For this review, take the finished solid that the model builds, in its own axes (mm). A direction names the side the tool comes from. Give positions to 0.01 mm unless a question says otherwise; leave off trailing zeros. Loops run counter-clockwise (first coordinate to the right, second up) from the corner with the lowest first, then second, coordinate; pieces in that order, holes last.
```python
from build123d import *

# Parameters (mm, degrees)
F0_W     = 12.7
F0_H     = 12.7
F1_DEPTH = 12.7
F2_DEPTH = 25.4
F3_W     = 12.9194361269
F3_H     = 12.7
F4_DEPTH = 12.7
F5_W     = 12.7
F5_H     = 12.7
F6_DEPTH = 12.7
F7_W     = 12.7
F7_H     = 12.7
F8_DEPTH = 12.7
F9_T     = -2.54


with BuildPart() as f1:
    # F0 (on Front) → F1 (new body)
    with BuildSketch(Plane.XZ):
        with Locations((0.4788246006, 3.6696097578)):
            Rectangle(F0_W, F0_H)
    extrude(amount=F1_DEPTH)

    # F2 (add): a face of the model
    f2_faces = [f1.faces().sort_by_distance(p)[0] for p in [
        (6.8288246006, -6.35, 3.6696097578),
    ]]
    extrude(f2_faces, amount=F2_DEPTH)

    # F3 (on face) → F4 (join)
    with BuildSketch(Plane(origin=(0, 0, 0), x_dir=(-1, 0, 0), z_dir=(0, 1, 0))):
        with Locations((-25.7691065371, 3.6696097578)):
            Rectangle(F3_W, F3_H)
    extrude(amount=F4_DEPTH)

    # F5 (on face) → F6 (join)
    with BuildSketch(Plane(origin=(0, 0, 0), x_dir=(-1, 0, 0), z_dir=(0, 1, 0))):
        with Locations((-0.4788246006, 3.6696097578)):
            Rectangle(F5_W, F5_H)
    extrude(amount=F6_DEPTH)

    # F7 (on face) → F8 (join)
    with BuildSketch(Plane.XY.offset(10.0196097578)):
        with Locations((0.4788246006, -6.35)):
            Rectangle(F7_W, F7_H)
    extrude(amount=F8_DEPTH)

    # F9 (hollow: no face is removed)
    offset(amount=F9_T, kind=Kind.INTERSECTION, mode=Mode.SUBTRACT)


solid = f1.part
```
Item 1: Take a section at B-B on z = 17.5. Give the boundary of the cut face in (x, y), and give its area (3 significant figures).
Answer:
outline: (-5.87, -12.7) - (6.83, -12.7) - (6.83, 0) - (-5.87, 0) - close; hole (-3.33, -10.16) - (4.29, -10.16) - (4.29, -2.54) - (-3.33, -2.54) - close
area: 103 mm2
Item 2: Clearance check with flat-ended pins moving along their axes: pin 1 Ø3.5 at (x, z) = (15, 1) entering from +Y; pin 2 Ø4 at (y, z) = (-8, 19.5) entering from +X. State where each tip first meets the part, or that it passes through.
Answer:
pin 1: stops at y = 0
pin 2: stops at x = 6.83
Item 3: Tool access review of faces 1 (the flat face through (-5.871, -3, 7)), 2 (the flat face through (1, 6, 10.02)), 3 (the flat face through (19.309, 6, 4)), 4 (the flat face through (29.689, 0, 4)): name each direction out of +Z, -Z, +X, -X, +Y, -Y from which nothing blocks a thin tool from reaching the whole face with its end or side.
Answer:
face 1: +Z, -Z, -X, +Y, -Y
face 2: +Z, +X, -X, +Y
face 3: +Z, -Z, +Y
face 4: none
Item 4: For L1, parallel to X at y = 4.75, z = 7.25; L2, parallel to Y at x = -2, z = 9; L3, parallel to Y at x = -1, z = 6.5, list the stretches that pass through material, from the lowest coordinate up.
Answer:
L1: x = -5.87 to -3.33, 4.29 to 6.83, 19.31 to 21.85, 29.69 to 32.23
L2: y = -12.7 to -10.16, -2.54 to 12.7
L3: y = -12.7 to -10.16, 10.16 to 12.7
Item 5: The part is to be moulded in two halves that separate along Y. For faces 5 (the flat face through (6.829, 6, 4)), 6 (the flat face through (4.289, 4, 4)), 7 (the flat face through (0, 0, 16)), 8 (the flat face through (9, -10.16, 5)), say which applies: released by +Y, released by -Y, zero draft, split by the parting line, or undercut.
Answer:
face 5: zero draft
face 6: undercut
face 7: released by +Y
face 8: undercut
Item 6: Take a section at A-A on y = 1. Give the boundary of the cut face in (x, z).
Answer:
outline: (-5.87, -2.68) - (6.83, -2.68) - (6.83, 10.02) - (-5.87, 10.02) - close; (19.31, -2.68) - (32.23, -2.68) - (32.23, 10.02) - (19.31, 10.02) - close; hole (-3.33, -0.14) - (4.29, -0.14) - (4.29, 7.48) - (-3.33, 7.48) - close; hole (21.85, -0.14) - (29.69, -0.14) - (29.69, 7.48) - (21.85, 7.48) - close
Item 7: Take a section at C-C on y = -2. Give the boundary of the cut face in (x, z).
Answer:
outline: (-5.87, -2.68) - (32.23, -2.68) - (32.23, 10.02) - (6.83, 10.02) - (6.83, 22.72) - (-5.87, 22.72) - close; hole (-3.33, -0.14) - (4.29, -0.14) - (4.29, 7.48) - (-3.33, 7.48) - close; hole (21.85, -0.14) - (29.69, -0.14) - (29.69, 7.48) - (21.85, 7.48) - close
Item 8: Take a section at D-D on x = 24. Give the boundary of the cut face in (y, z), and give its area (3 significant figures).
Answer:
outline: (-12.7, -2.68) - (12.7, -2.68) - (12.7, 10.02) - (-12.7, 10.02) - close; hole (-10.16, -0.14) - (10.16, -0.14) - (10.16, 7.48) - (-10.16, 7.48) - close
area: 168 mm2
